CAD build for the part. Positions are in the model's coordinates, mm. A direction names the side the tool comes from. Round coordinates to 2 decimals unless told otherwise and drop trailing zeros. Order: outer loops, then holes, each group sorted by start corner. A loop starts at its lowest first (then second) coordinate and runs counter-clockwise, first axis right, second up. Notation, with made-up numbers: (11.5, 50) - (64.5, 50) arc R17 ccw to (64.5, 66) - close; hole circle Ø8 at (-17, 59.25). An arc over 180 degrees is marked (long way). Write item = value, one per line.
Autodesk Inventor part; units mm, degrees
ref_plane "YZ Plane" through (0, 0, 0) normal (1, 0, 0) x (0, 1, 0)
ref_plane "XZ Plane" through (0, 0, 0) normal (0, 1, 0) x (-1, 0, 0)
ref_plane "XY Plane" through (0, 0, 0) normal (0, 0, 1) x (1, 0, 0)
sketch "Sketch1" plane through (0, 0, 0) normal (0, 0, 1) x (1, 0, 0)
  line L0 (0, 277.6336) -> (196.3166, 196.3166) construction
  line L1 (196.3166, 196.3166) -> (277.6336, 0) construction
  line L2 (277.6336, 0) -> (196.3166, -196.3166) construction
  line L3 (196.3166, -196.3166) -> (0, -277.6336) construction
  line L4 (0, -277.6336) -> (-196.3166, -196.3166) construction
  line L5 (-196.3166, -196.3166) -> (-277.6336, 0) construction
  line L6 (-277.6336, 0) -> (-196.3166, 196.3166) construction
  line L7 (-196.3166, 196.3166) -> (0, 277.6336)
  line L8 (-196.3166, 196.3166) -> (0, 277.6336)
  line L9 (-461.2666, 773.8898) -> (-221.0579, 873.3874)
  line L10 (-98.1583, 236.9751) -> (-341.1623, 823.6386) construction
  line L11 (-221.0579, 873.3874) -> (0, 873.3874)
  line L12 (0, 873.3874) -> (0, 277.6336)
  line L13 (-461.2666, 773.8898) -> (-617.5782, 617.5782)
  line L14 (-617.5782, 617.5782) -> (-196.3166, 196.3166)
  point P0 (0, 0)
  point P1 (0, 0)
  dimension "d0" = 513
  dimension "d2" = 260
  dimension "d3" = 635
extrude "Extrusion1" add sketch "Sketch1" along normal mid plane 8
sketch "Sketch2" plane through (0, 0, 4) normal (0, 0, 1) x (1, 0, 0)
  line L0 (-221.0579, 873.3874) -> (-461.2666, 773.8898)
  line L1 (-461.2666, 773.8898) -> (-617.5782, 617.5782)
  line L2 (-236.3886, 531.4957) -> (-415.0608, 457.4872)
  line L3 (-196.3166, 196.3166) -> (0, 277.6336)
  line L4 (-98.1583, 236.9751) -> (-341.1623, 823.6386) construction
  line L5 (-617.5782, 617.5782) -> (-196.3166, 196.3166)
  line L6 (-415.0608, 457.4872) -> (-575.1518, 617.5782)
  line L7 (-575.1518, 617.5782) -> (-444.273, 748.457)
  line L8 (-444.273, 748.457) -> (-343.54, 790.182)
  line L9 (-236.3886, 531.4957) -> (-343.54, 790.182)
  line L10 (-208.6722, 542.9762) -> (-30, 616.9847)
  line L11 (-30, 616.9847) -> (-30, 843.3874)
  line L12 (-30, 843.3874) -> (-215.0906, 843.3874)
  line L13 (-215.0906, 843.3874) -> (-315.8236, 801.6625)
  line L14 (-208.6722, 542.9762) -> (-315.8236, 801.6625)
  line L15 (0, 277.6336) -> (0, 873.3874)
  line L16 (-415.0608, 457.4872) -> (-30, 616.9847) construction
  line L17 (-392.0998, 434.5262) -> (-30, 584.5129)
  line L18 (-189.2776, 231.704) -> (-30, 297.679)
  line L19 (-30, 297.679) -> (-30, 584.5129)
  line L20 (-189.2776, 231.704) -> (-392.0998, 434.5262)
  point P0 (0, 0)
  dimension "d11" = 30
  dimension "d12" = 280
  dimension "d13" = 30
  dimension "d14" = 30
  dimension "d15" = 15
  dimension "d21" = 30
  dimension "d22" = 30
  dimension "d23" = 30
  dimension "d24" = 30
extrude "Extrusion2" cut sketch "Sketch2" against normal up to surface (8 mm away)
fillet "Fillet1" radius 10 12 edges at (-575.1518, 617.5782, 0) (-343.54, 790.182, 0) (-236.3886, 531.4957, 0) (-415.0608, 457.4872, 0) (-315.8236, 801.6625, 0) (-30, 843.3874, 0) (-30, 616.9847, 0) (-208.6722, 542.9762, 0) (-392.0998, 434.5262, 0) (-30, 584.5129, 0) (-30, 297.679, 0) (-189.2776, 231.704, 0)
sketch "Sketch5" plane through (0, 0, 4) normal (0, 0, 1) x (1, 0, 0)
  line L0 (-221.0579, 873.3874) -> (-461.2666, 773.8898)
  line L1 (0, 873.3874) -> (-221.0579, 873.3874)
  line L2 (-461.2666, 773.8898) -> (-617.5782, 617.5782)
  line L3 (-617.5782, 617.5782) -> (-196.3166, 196.3166)
  line L4 (-196.3166, 196.3166) -> (0, 277.6336)
  line L5 (0, 277.6336) -> (0, 873.3874)
  line L6 (-15, 858.3874) -> (-218.0743, 858.3874) construction
  line L7 (-218.0743, 858.3874) -> (-452.7698, 761.1734) construction
  line L8 (-452.7698, 761.1734) -> (-596.365, 617.5782) construction
  line L9 (-596.365, 617.5782) -> (-192.7971, 214.0103) construction
  line L10 (-192.7971, 214.0103) -> (-15, 287.6563) construction
  line L11 (-15, 287.6563) -> (-15, 858.3874) construction
  line L12 (-378.273, 440.2535) -> (-43.8268, 578.7856)
  line L13 (-212.4991, 552.215) -> (-311.9967, 792.4237)
  line L14 (-418.5803, 439.7935) -> (-15, 606.962) construction
  line L15 (-216.7902, 523.3778) -> (-335.422, 809.7804) construction
  circle A0 centre (-335.422, 809.7804) radius 2
  circle A1 centre (-216.7902, 523.3778) radius 2
  circle A2 centre (-295.8793, 714.3159) radius 2
  circle A3 centre (-256.3367, 618.8515) radius 2
  circle A4 centre (-596.365, 617.5782) radius 2
  circle A5 centre (-515.5729, 536.7861) radius 2
  circle A6 centre (-434.7809, 455.9941) radius 2
  circle A7 centre (-353.9889, 375.2021) radius 2
  circle A8 centre (-273.1968, 294.41) radius 2
  circle A9 centre (-192.4048, 213.618) radius 2
  circle A10 centre (-317.0311, 481.8566) radius 2
  circle A11 centre (-103.8986, 250.8333) radius 2
  circle A12 centre (-518.5832, 695.3599) radius 2
  circle A13 centre (-437.0488, 767.6852) radius 2
  circle A14 centre (-15, 858.3874) radius 2
  circle A15 centre (-15, 744.1302) radius 2
  circle A16 centre (-15, 629.873) radius 2
  circle A17 centre (-15, 515.6158) radius 2
  circle A18 centre (-15, 401.3586) radius 2
  circle A19 centre (-15, 287.1014) radius 2
  circle A20 centre (-116.5492, 564.8989) radius 2
  circle A21 centre (-125, 858.3874) radius 2
  circle A22 centre (-233.7953, 851.8756) radius 2
  point P0 (0, 0)
  dimension "d32" = 15
  dimension "d33" = 15
  dimension "d34" = 15
  dimension "d35" = 4
  dimension "d37" = 103.33
  dimension "d38" = 103.33
  dimension "d43" = 114.2572
  dimension "d49" = 108.5
  dimension "d50" = 110
  dimension "d51" = 110
extrude "Extrusion4" cut sketch "Sketch5" against normal up to surface (8 mm away) contours A0 | A1 | A2 | A3 | A4 | A5 | A6 | A7 | A8 | A9 | A10 | A11 | A12 | A13 | A14 | A15 | A16 | A17 | A18 | A19 | A20 | A21 | A22
equation "\"d0\" = Барабан_габарит_по_кассетам"
equation "\"d2\" = Кассета_длина_грани"
equation "\"d3\" = Кассета_высота"
equation "\"d11\" = d13"
equation "\"d14\" = d13"
equation "\"d15\" = 0.5 * d13"
equation "\"d21\" = d13"
equation "\"d22\" = d13"
equation "\"d23\" = d13"
equation "\"d24\" = d13"
properties part number "ДМФ 01 56 Крепление сетки к кассете"
(1) Band-saw the part on D-D on z = 1. Count the separate pieces of the cut face and the enclosed holes in it, plus the area to 3 significant figures.
Solved:
separate_pieces = 1
enclosed_holes = 26
area = 80,300 mm²
(2) Pull direction Y, two halves, no side cores. Call faces 1 (the flat face through (-213.39, 508.55, 0.06)), 2 (the flat face through (-342.844, 822.942, -0.056)), 3 (the flat face through (-326.11, 494.33, 0.06)), 4 (the flat face through (-242, 562, -4)): released by +Y, released by -Y, zero draft, split by the parting line, or undercut.
Solved:
face_1 = undercut
face_2 = released by +Y
face_3 = undercut
face_4 = zero draft
(3) Band-saw the part on C-C on y = 269.5. List the corners of the cut face in (x, z), plus the area to 3 significant figures.
Solved:
outline = (-269.5, -4) - (-227.07, -4) - (-227.07, 4) - (-269.5, 4) - close; (-98.03, -4) - (-19.64, -4) - (-19.64, 4) - (-98.03, 4) - close
area = 967 mm²
(4) Probe line 1 along Y through (x, z) = (-75, 1.5); line 2 along Y through (x, z) = (-200, 2.25); line 3 along X through (y, z) = (588, 0.75). List the from-to ranges inside material, lowest first.
Solved:
line_1 = 246.57 to 279.04, 565.87 to 598.35, 843.39 to 873.39
line_2 = 200 to 242.43, 514.1 to 546.59, 843.39 to 873.39
line_3 = -588 to -545.57, -259.79 to -227.32, -99.98 to 0
(5) Tool access for faces 5 (the flat face through (-538.328, 696.828, -0.056)), 6 (the flat face through (-261.551, 670.638, 0.056)): list every direction of +Z, -Z, +X, -X, +Y, -Y with a clear straight run to the whole face (end or side of a thin tool).
Solved:
face_5 = +Z, -Z, -X, +Y
face_6 = +Z, -Z
(6) Band-saw the part on A-A on y = 725. List the corners of the cut face in (x, z), plus the area to 3 significant figures.
Solved:
outline = (-510.16, -4) - (-467.73, -4) - (-467.73, 4) - (-510.16, 4) - close; (-316.54, -4) - (-284.07, -4) - (-284.07, 4) - (-316.54, 4) - close; (-30, -4) - (0, -4) - (0, 4) - (-30, 4) - close
area = 839 mm²
(7) Band-saw the part on B-B on x = -174. List the corners of the cut face in (y, z).
Solved:
outline = (205.56, -4) - (238.03, -4) - (238.03, 4) - (205.56, 4) - close; (524.87, -4) - (557.34, -4) - (557.34, 4) - (524.87, 4) - close; (843.39, -4) - (873.39, -4) - (873.39, 4) - (843.39, 4) - close
(8) Drop flat-ended pins along their axis: pin 1 (4 mm diameter, centred on x = -110, z = -0.5, fed in from -Y); pin 2 (1 mm diameter, centred on x = -438.5, z = 0.5, fed in from -Y). Give the stop position or say it passes through.
Solved:
pin_1 = 231.24
pin_2 = 438
